The listing builds one solid part. Answer for the finished solid, in the listing's coordinates (mm). Face numbers are marked on the shaded views. A direction names the side the tool comes from. Give positions to 0.01 mm unless a question says otherwise; leave off trailing zeros. Order: outer loops, then holes, each group sorted by start corner. A loop starts at its lowest first (then second) coordinate and runs counter-clockwise, first axis right, second up. Notation, with made-up numbers: (19.5, 70) - (49.5, 70) arc R20 ccw to (49.5, 96) - close; hole circle Ø6 at (72.25, 35.5). An arc over 180 degrees is marked (long way). Answer as CSV lines item,"result". Start each with the question number.
1. Consider line 1 along Y through (x, z) = (0.25, 2.15); line 2 along X through (y, z) = (-13, 1.7); line 3 along Y through (x, z) = (-1.5, 2.8). Determine where each line is inside the solid, lowest interval first. Write a range as [from, to].
2. Determine the mould class of the marked faces 1, 2 and 3 for opening direction X: +X half, -X half, draft (parallel to the pull), parting line (faces both ways), or undercut.
3. Flat-ended cylindrical pins translate along their axes: pin 1 (1.2 mm diameter, centred on x = 5.5, z = 1, fed in from -Y); pin 2 (1.5 mm diameter, centred on x = -1, z = 0.5, fed in from -Y). Find the tip coordinate at first contact, or state that the pin passes through.
4. Which of the six approach directions +Z, -Z, +X, -X, +Y, -Y give full straight-line access (tool end or side, diameter ignored) to the marked faces 4, 5 and 6?
5. Section D-D on y = -6.75 is taken. Give the vertices of the cut face in (x, z), and give its area (3 significant figures).
6. Section C-C on y = 0.25 is taken. Give the vertices of the cut face in (x, z).
7. Section A-A on z = 2.5 is taken. Give the vertices of the cut face in (x, y), and give its area (3 significant figures).
8. Section B-B on x = 0.25 is taken. Give the vertices of the cut face in (y, z).
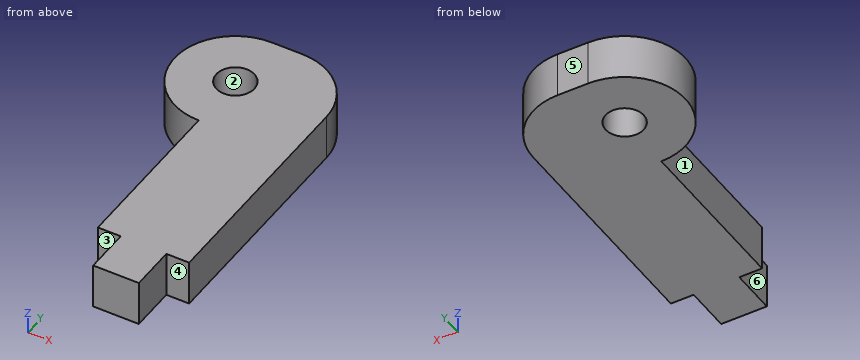
from build123d import *

# Parameters (mm, degrees)
SKETCH2_R           = 1.25
BOSS_EXTRUDE1_DEPTH = 3
FILLET1_R           = 4


with BuildPart() as part:
    # Sketch2 → Boss-Extrude1 (new body)
    with BuildSketch(Plane.XY):
        with BuildLine():
            Line((6, 4), (6, -15))
            Line((6, -15), (4.5, -15))
            Line((4.5, -15), (4.5, -18))
            Line((4.5, -18), (1.5, -18))
            Line((1.5, -18), (1.5, -15))
            Line((1.5, -15), (0, -15))
            Line((0, -15), (0, -4))
            ThreePointArc((0, -4), (-4, 0), (0, 4))
            Line((0, 4), (6, 4))
        make_face()
        Circle(SKETCH2_R, mode=Mode.SUBTRACT)
    extrude(amount=BOSS_EXTRUDE1_DEPTH)

    # Fillet1
    fillet1_edges = [part.edges().sort_by_distance(p)[0] for p in [
        (6, 4, 1.5),
    ]]
    fillet(fillet1_edges, radius=FILLET1_R)


solid = part.part
Checks:
1,line 1,"y = [-15, -1.22], [1.22, 4]"
1,line 2,"x = [0, 6]"
1,line 3,"y = [-3.71, 3.71]"
2,face 1,"-X half"
2,face 2,"undercut"
2,face 3,"draft"
3,pin 1,"stops at y = -15"
3,pin 2,"stops at y = -3.99"
4,face 4,"+Z, -Z, +X, -Y"
4,face 5,"+Z, -Z, +X, -X, +Y"
4,face 6,"+Z, -Z, -X, -Y"
5,outline,"(0, 0) - (6, 0) - (6, 3) - (0, 3) - close"
5,area,"18.0 mm²"
6,outline,"(-3.99, 0) - (-1.22, 0) - (-1.22, 3) - (-3.99, 3) - close; (1.22, 0) - (5.99, 0) - (5.99, 3) - (1.22, 3) - close"
7,outline,"(0, -15) - (1.5, -15) - (1.5, -18) - (4.5, -18) - (4.5, -15) - (6, -15) - (6, 0) arc R4 ccw to (2, 4) - (0, 4) arc R4 ccw to (0, -4) - close; hole circle Ø2.5 at (0, 0)"
7,area,"140 mm²"
8,outline,"(-15, 0) - (-1.22, 0) - (-1.22, 3) - (-15, 3) - close; (1.22, 0) - (4, 0) - (4, 3) - (1.22, 3) - close"
